Here's how the part is built. I have some questions about the finished solid (model axes, mm). Face numbers are marked on the shaded views. A direction names the side the tool comes from. Coordinates: 2 decimals unless noted, no trailing zeros. Order: outer loops, then holes, each group sorted by start corner. A loop starts at its lowest first (then second) coordinate and runs counter-clockwise, first axis right, second up. Notation, with made-up numbers: (78, 4.5) - (120, 4.5) arc R21 cw to (120, 21.5) - close; hole circle Ø6 at (33, 58.5). An arc over 180 degrees is marked (long way). Answer in a Markdown table with one row per item. Add a question column.
Item 1: I want a section at A-A (x = -3). Please give me the cut outline in (y, z).
Item 2: On a 3-axis mill with a long thin cutter (end or side, diameter ignored), from which of +Z, -Z, +X, -X, +Y, -Y can I reach the whole of each face in a straight line? I mean the marked faces 1 and 2. Say none if no direction works.
Item 3: Will these pins go through, and if not, where does the flat tip stop? pin 1 Ø2.5 at (y, z) = (12, 35.5) entering from +X; pin 2 Ø1.8 at (y, z) = (12.41, 17.6) entering from +X; pin 3 Ø8 at (x, y) = (-20.5, -13) entering from +Z; pin 4 Ø0.9 at (x, y) = (55, 10.5) entering from +Z.
Item 4: Thinking about a two-plate mould opening in Y: for the marked faces 3, 4, 5 and 6, which applies, +Y half, -Y half, draft (parallel to the pull), parting line (faces both ways), or undercut?
Item 5: If I drill on line 1 along Y through (x, z) = (58.9, 17.6); line 2 along X through (y, z) = (15, 34.5); line 3 along Y through (x, z) = (-52, 37), over which ranges is the centre line in solid material (lowest first)? Write a range as from..to.
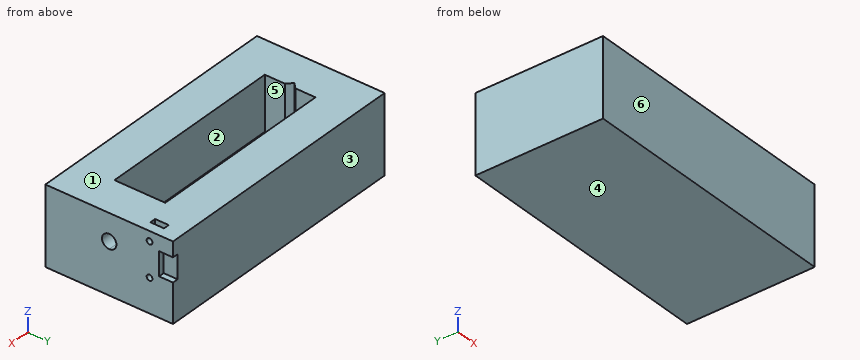
```python
from build123d import *

# Parameters (mm, degrees)
F0_W      = 138
F0_H      = 66.4
F1_DEPTH  = 12.5
F2_W      = 20
F2_H      = 26.4
F3_DEPTH  = 28
F5_DEPTH  = 25
F7_DEPTH  = 3
F9_DEPTH  = 20
F10_DEPTH = 15
F8_W      = 3.067044
F8_H      = 3.546548
F11_DEPTH = 30


with BuildPart() as f1:
    # F0 (on Top) → F1 (new body)
    with BuildSketch(Plane.XY):
        with Locations((-7.109798, -8.569356)):
            Rectangle(F0_W, F0_H)
    extrude(amount=F1_DEPTH)

    # F2 (on face) → F3 (join)
    with BuildSketch(Plane.XY.offset(12.5)):
        Polygon((-76.109798, -21.769356), (-76.109798, -41.769356), (61.890202, -41.769356), (61.890202, -21.769356), (41.890202, -21.769356), (-56.109798, -21.769356), (-58.859691, -21.769356), align=None)
        Polygon((-76.109798, 4.630644), (-76.109798, -21.769356), (-58.859691, -21.769356), (-58.859691, -8.569356), (-58.859691, 4.630644), align=None)
        with Locations((51.890202, -8.569356)):
            Rectangle(F2_W, F2_H)
        Polygon((-76.109798, 24.630644), (-76.109798, 4.630644), (-58.859691, 4.630644), (-56.109798, 4.630644), (41.890202, 4.630644), (61.890202, 4.630644), (61.890202, 24.630644), align=None)
        Polygon((-58.859691, 4.630644), (-58.859691, -8.569356), (-56.109798, -5.819463), (-56.109798, 4.630644), align=None)
        Polygon((-58.859691, -8.569356), (-58.859691, -21.769356), (-56.109798, -21.769356), (-56.109798, -11.319249), align=None)
    extrude(amount=F3_DEPTH)

    # F4 (on face) → F5 (cut)
    with BuildSketch(Plane.YZ.offset(61.890202)):
        with BuildLine():
            ThreePointArc((-8.569356, 22.75), (-5.917706, 23.84835), (-4.819356, 26.5))
            ThreePointArc((-4.819356, 26.5), (-5.917706, 29.15165), (-8.569356, 30.25))
            Line((-8.569356, 30.25), (-8.569356, 22.75))
        make_face()
        with BuildLine():
            Line((-8.569356, 22.75), (-8.569356, 30.25))
            ThreePointArc((-8.569356, 30.25), (-12.319356, 26.5), (-8.569356, 22.75))
        make_face()
    extrude(amount=-F5_DEPTH, mode=Mode.SUBTRACT)

    # F6 (on face) → F7 (cut)
    with BuildSketch(Plane.YZ.offset(61.890202)):
        Polygon((17.405644, 32.680817), (17.405644, 26.5), (17.405644, 20.319183), (24.630644, 20.319183), (24.630644, 32.680817), align=None)
    extrude(amount=-F7_DEPTH, mode=Mode.SUBTRACT)

    # F6 (on face) → F9 (cut)
    with BuildSketch(Plane.YZ.offset(61.890202)):
        with BuildLine():
            ThreePointArc((13.905644, 17.6), (13.466304, 18.66066), (12.405644, 19.1))
            ThreePointArc((12.405644, 19.1), (11.344984, 16.53934), (13.905644, 17.6))
        make_face()
        with BuildLine():
            Line((12.405644, 35.4), (12.405644, 36.9))
            ThreePointArc((12.405644, 36.9), (10.905644, 35.4), (12.405644, 33.9))
            Line((12.405644, 33.9), (12.405644, 35.4))
        make_face()
        with BuildLine():
            ThreePointArc((12.405644, 33.9), (13.466304, 34.33934), (13.905644, 35.4))
            ThreePointArc((13.905644, 35.4), (13.466304, 36.46066), (12.405644, 36.9))
            Line((12.405644, 36.9), (12.405644, 35.4))
            Line((12.405644, 35.4), (12.405644, 33.9))
        make_face()
    extrude(amount=-F9_DEPTH, mode=Mode.SUBTRACT)

    # F6 (on face) → F10 (cut)
    with BuildSketch(Plane.YZ.offset(61.890202)):
        with BuildLine():
            ThreePointArc((12.405644, 33.9), (13.466304, 34.33934), (13.905644, 35.4))
            ThreePointArc((13.905644, 35.4), (13.466304, 36.46066), (12.405644, 36.9))
            Line((12.405644, 36.9), (12.405644, 35.4))
            Line((12.405644, 35.4), (12.405644, 33.9))
        make_face()
        with BuildLine():
            Line((12.405644, 35.4), (12.405644, 36.9))
            ThreePointArc((12.405644, 36.9), (10.905644, 35.4), (12.405644, 33.9))
            Line((12.405644, 33.9), (12.405644, 35.4))
        make_face()
        with BuildLine():
            ThreePointArc((13.905644, 17.6), (13.466304, 18.66066), (12.405644, 19.1))
            ThreePointArc((12.405644, 19.1), (11.344984, 16.53934), (13.905644, 17.6))
        make_face()
    extrude(amount=-F10_DEPTH, mode=Mode.SUBTRACT)

    # F8 (on face) → F11 (cut)
    with BuildSketch(Plane.XY.offset(40.5)):
        with Locations((55.204206, 10.50737)):
            Rectangle(F8_W, F8_H)
        with Locations((55.204206, 14.053918)):
            Rectangle(F8_W, F8_H)
    extrude(amount=-F11_DEPTH, mode=Mode.SUBTRACT)


solid = f1.part
```
Values follow:
| question | item | result |
|---|---|---|
| 1 | outline | (-41.77, 0) - (24.63, 0) - (24.63, 40.5) - (4.63, 40.5) - (4.63, 12.5) - (-21.77, 12.5) - (-21.77, 40.5) - (-41.77, 40.5) - close |
| 2 | face 1 | +Z, +X, -X, +Y, -Y |
| 2 | face 2 | +Z |
| 3 | pin 1 | stops at x = 61.89 |
| 3 | pin 2 | stops at x = 41.89 |
| 3 | pin 3 | stops at z = 12.5 |
| 3 | pin 4 | stops at z = 10.5 |
| 4 | face 3 | +Y half |
| 4 | face 4 | draft |
| 4 | face 5 | undercut |
| 4 | face 6 | -Y half |
| 5 | line 1 | y = -41.77..10.91, 13.91..24.63 |
| 5 | line 2 | x = -76.11..53.67, 56.74..61.89 |
| 5 | line 3 | y = -41.77..-21.77, 4.63..24.63 |
